Build history of the part. All positions in model axes, mm. Face numbers are marked on the shaded views. A direction names the side the tool comes from. Give positions to 0.01 mm unless a question says otherwise; leave off trailing zeros. Order: outer loops, then holes, each group sorted by start corner. A loop starts at its lowest first (then second) coordinate and runs counter-clockwise, first axis right, second up. Notation, with made-up numbers: (72, 5) - (113, 5) arc R26 cw to (113, 29) - close; hole circle Ø3 at (66.25, 13). An arc over 180 degrees is marked (long way). Use a Markdown table: item, result.
from build123d import *

# Parameters (mm, degrees)
F0_R   = 2
F0_R_2 = 1.3


with BuildPart() as f2:
    # F2: sweep along a path in F1
    with BuildLine(Plane.YZ) as f2_path:
        Line((0, 0), (0, 44))
        ThreePointArc((0, 44), (-4.686291501, 55.313708499), (-16, 60))
        Line((-16, 60), (-100, 60))
    # F0 (on Top) → F2 (sweep)
    with BuildSketch(Plane.XY):
        Circle(F0_R)
        Circle(F0_R_2, mode=Mode.SUBTRACT)
    sweep(path=f2_path.line)


solid = f2.part
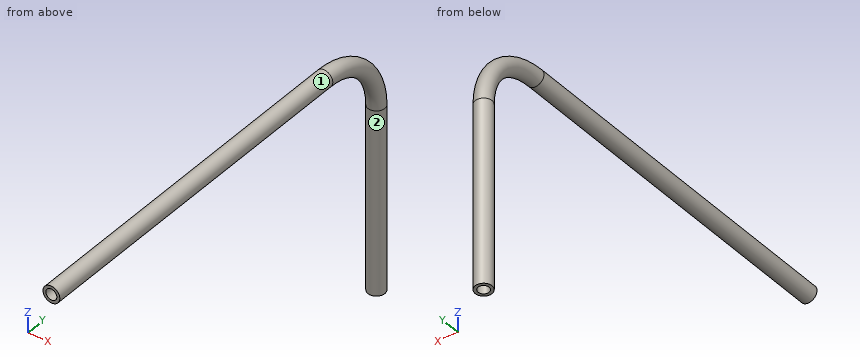
1) Wall check: line 1 (Y direction, x = 0.1, z = 18); line 2 (Z direction, x = 0, y = -72). Give the ranges that are in metal, low to high. Write a range as from..to.
Computed:
| item | result |
|---|---|
| line 1 | y = -2..-1.3, 1.3..2 |
| line 2 | z = 58..58.7, 61.3..62 |
2) Slice it at C-C (y = -48). Write the cut outline in (x, z), and give its area (3 significant figures).
Computed:
| item | result |
|---|---|
| outline | circle Ø4 at (0, 60); hole circle Ø2.6 at (0, 60) |
| area | 7.26 mm² |
3) Slice it at A-A (x = 0). Write the cut outline in (y, z).
Computed:
| item | result |
|---|---|
| outline | (-100, 58) - (-16, 58) arc R14 cw to (-2, 44) - (-2, 0) - (-1.3, 0) - (-1.3, 44) arc R14.7 ccw to (-16, 58.7) - (-100, 58.7) - close; (-100, 61.3) - (-16, 61.3) arc R17.3 cw to (1.3, 44) - (1.3, 0) - (2, 0) - (2, 44) arc R18 ccw to (-16, 62) - (-100, 62) - close |
4) Tool access for the marked faces 1 and 2: list every direction of +Z, -Z, +X, -X, +Y, -Y with a clear straight run to the whole face (end or side of a thin tool).
Computed:
| item | result |
|---|---|
| face 1 | -Y |
| face 2 | -Z |
5) Slice it at B-B (z = 33). Write the cut outline in (x, y), and give its area (3 significant figures).
Computed:
| item | result |
|---|---|
| outline | circle Ø4 at (0, 0); hole circle Ø2.6 at (0, 0) |
| area | 7.26 mm² |
6) Pin check, flat tips, straight feed: P1, Ø1.5, axis at x = 1.5, z = 55.5, coming from the -Y side; P2, Ø2, axis at x = -0.5, z = 24, coming from the -Y side; P3, Ø1, axis at x = 0.5, y = -67, coming from the -Z side. Stop position of each tip, or through.
Computed:
| item | result |
|---|---|
| P1 | stops at y = -8.38 |
| P2 | stops at y = -2 |
| P3 | stops at z = 58 |
